Model file for the job. Use its own axes, mm. A direction names the side the tool comes from. Give positions to 0.01 mm unless a question says otherwise; leave off trailing zeros. Loops run counter-clockwise (first coordinate to the right, second up) from the corner with the lowest first, then second, coordinate; pieces in that order, holes last. Notation, with made-up numbers: (23, 89) - (58, 89) arc R6 ccw to (58, 94) - close; hole circle Ø11 at (65.5, 88.25). An arc over 180 degrees is marked (long way). Use a Markdown table: item, result.
from build123d import *

# Parameters (mm, degrees)
BOSS_EXTRUDE5_DEPTH = 80.682375276
SKETCH6_R           = 7.713097058
CUT_EXTRUDE3_DEPTH  = 25
SKETCH7_R           = 3.5
CUT_EXTRUDE4_DEPTH  = 5
SKETCH8_R           = 7.713097058
CUT_EXTRUDE5_DEPTH  = 50
SKETCH9_R           = 3.5
CUT_EXTRUDE6_DEPTH  = 50


with BuildPart() as part:
    # Sketch3 → Boss-Extrude5 (new body)
    with BuildSketch(Plane(origin=(0, 0, 0), x_dir=(0, 1, 0), z_dir=(0, 0, 1))):
        with BuildLine():
            Line((-12.5, 0), (-12.5, -12.5))
            Line((-12.5, -12.5), (12.5, -12.5))
            Line((12.5, -12.5), (12.5, 0))
            ThreePointArc((12.5, 0), (0, 12.5), (-12.5, 0))
        make_face()
    extrude(amount=BOSS_EXTRUDE5_DEPTH)

    # Sketch6 → Cut-Extrude3 (cut)
    with BuildSketch(Plane.XY.offset(80.682375276)):
        Circle(SKETCH6_R)
    extrude(amount=-CUT_EXTRUDE3_DEPTH, mode=Mode.SUBTRACT)

    # Sketch7 → Cut-Extrude4 (cut)
    with BuildSketch(Plane(origin=(0, 0, 0), x_dir=(1, 0, 0), z_dir=(0, 0, -1))):
        with Locations(Location((0, 0, 0), (0, 0, 180))):
            Circle(SKETCH7_R)
    extrude(amount=-CUT_EXTRUDE4_DEPTH, mode=Mode.SUBTRACT)

    # Sketch8 → Cut-Extrude5 (cut)
    with BuildSketch(Plane.XY.offset(55.682375276)):
        Circle(SKETCH8_R)
    extrude(amount=-CUT_EXTRUDE5_DEPTH, mode=Mode.SUBTRACT)

    # Sketch9 → Cut-Extrude6 (cut)
    with BuildSketch(Plane(origin=(0, 0, 0), x_dir=(1, 0, 0), z_dir=(0, 0, -1))):
        with Locations(Location((0, 0, 0), (0, 0, 180))):
            Circle(SKETCH9_R)
    extrude(amount=-CUT_EXTRUDE6_DEPTH, mode=Mode.SUBTRACT)


solid = part.part
(1) Slice it at C-C, the plane x = 6. Write the cut outline in (y, z).
Computed:
| item | result |
|---|---|
| outline | (-12.5, 0) - (12.5, 0) - (12.5, 80.68) - (4.85, 80.68) - (4.85, 5.68) - (-4.85, 5.68) - (-4.85, 80.68) - (-12.5, 80.68) - close |
(2) 3-axis set-ups, long thin cutter, end or side, ignore diameter. For faces 5 (the flat face through (12.5, 0, 40)), 6 (the flat face through (3.3, -1.6, 5.682)): which of +Z, -Z, +X, -X, +Y, -Y reach the whole face in a straight line?
Computed:
| item | result |
|---|---|
| face 5 | +Z, -Z, +X, +Y, -Y |
| face 6 | +Z |
(3) Drill centre lines: probe 1 along Y at (x, z) = (0, 4.45); probe 2 along X at (y, z) = (-0.5, 70.5); probe 3 along Y at (x, z) = (0, 35.5). Where is each one in solid material? Low to high. Write a range as [from, to].
Computed:
| item | result |
|---|---|
| probe 1 | [-12.5, -3.5], [3.5, 12.5] |
| probe 2 | [-12.49, -7.7], [7.7, 12.5] |
| probe 3 | [-12.5, -7.71], [7.71, 12.5] |
(4) Pin check, flat tips, straight feed: P1, Ø12.5, axis at x = 0, y = 0, coming from the -Z side; P2, Ø2, axis at x = -9, z = 31.5, coming from the -Y side; P3, Ø4, axis at x = -9.5, z = 27.5, coming from the +Y side; P4, Ø1.5, axis at x = -3, z = 45.5, coming from the +Y side. Stop position of each tip, or through.
Computed:
| item | result |
|---|---|
| P1 | z = 0 |
| P2 | y = -9.6 |
| P3 | y = 10 |
| P4 | y = 12.3 |
(5) Mould opens along Y. For faces 1 (the cylindrical face through (-6.121, -4.693, 43.707)), 2 (the flat face through (8, 0, 80.682)), 3 (the flat face through (6, 12.5, 40)), 4 (the cylindrical face through (-12.497, 0.275, 39.776)) say: pulls with the +Y half, pulls with the -Y half, needs draft (parallel to the pull), parting line crosses it, or undercut.
Computed:
| item | result |
|---|---|
| face 1 | undercut |
| face 2 | needs draft |
| face 3 | pulls with the +Y half |
| face 4 | parting line crosses it |
(6) Slice it at D-D, the plane x = -6.5. Write the cut outline in (y, z).
Computed:
| item | result |
|---|---|
| outline | (-10.68, 0) - (10.68, 0) - (10.68, 80.68) - (4.15, 80.68) - (4.15, 5.68) - (-4.15, 5.68) - (-4.15, 80.68) - (-10.68, 80.68) - close |
(7) Slice it at B-B, the plane z = 53.5. Write the cut outline in (x, y), plus the area to 3 significant figures.
Computed:
| item | result |
|---|---|
| outline | (0, -12.5) - (12.5, -12.5) - (12.5, 12.5) - (0, 12.5) arc R12.5 ccw to start; hole circle Ø15.43 at (0, 0) |
| area | 371 mm² |
(8) Slice it at A-A, the plane y = 0. Write the cut outline in (x, z), plus the area to 3 significant figures.
Computed:
| item | result |
|---|---|
| outline | (-12.5, 0) - (-3.5, 0) - (-3.5, 5.68) - (-7.71, 5.68) - (-7.71, 80.68) - (-12.5, 80.68) - close; (3.5, 0) - (12.5, 0) - (12.5, 80.68) - (7.71, 80.68) - (7.71, 5.68) - (3.5, 5.68) - close |
| area | 820 mm² |
